Solid Edge part; units mm, degrees
sketch "Sketch1" plane through (0, 0, 0) normal (0, 0, 1) x (1, 0, 0)
  line L0 (-12.5, -3) -> (12.5, -3)
  line L1 (12.5, -3) -> (12.5, 3)
  line L2 (12.5, 3) -> (-12.5, 3)
  line L3 (-12.5, 3) -> (-12.5, -3)
  dimension "D1" = 12.5
  dimension "D2" = 12.5
extrude "Protrusion1" add sketch "Sketch1" along normal blind 2
sketch "Sketch2" plane through (0, 0, 2) normal (0, 0, 1) x (1, 0, 0)
  line L0 (-12.5, 3) -> (12.5, 3)
  line L1 (12.5, 3) -> (12.5, 2)
  line L2 (12.5, 2) -> (-12.5, 2)
  line L3 (-12.5, 2) -> (-12.5, 3)
  line L4 (-12.5, -3) -> (12.5, -3)
  line L5 (12.5, -3) -> (12.5, -1)
  line L6 (12.5, -1) -> (-12.5, -1)
  line L7 (-12.5, -1) -> (-12.5, -3)
  dimension "D1" = 12.5
  dimension "D2" = 12.5
extrude "Extrusionsausprägung_2" add sketch "Sketch2" along normal blind 4
chamfer "Fase_1" distance 0.5 angle 45 3 edges at (0, -3, 6) (0, -1, 6) (0, 2, 6)
Model file for the job. Use its own axes, mm. A direction names the side the tool comes from. Give positions to 0.01 mm unless a question says otherwise; leave off trailing zeros. Write each loop counter-clockwise with the first axis right and the second up, starting at its lowest first coordinate (ties: lowest second). Pieces come first, ordered by that corner, then holes. Notation, with made-up numbers: M 64,41 L 82,41 A21 ccw 82,71 Z; hole C 7,89.25 d9. An arc over 180 degrees is marked long. Use a Markdown table: item, result.
1) Pin check, flat tips, straight feed: pin 1 (1.5 mm diameter, centred on x = 8, y = 2, fed in from -Z); pin 2 (1.5 mm diameter, centred on x = 5, y = 0.5, fed in from +Z). Stop position of each tip, or through.
Responses:
| item | result |
|---|---|
| pin 1 | stops at z = 0 |
| pin 2 | stops at z = 2 |
2) Cut at A-A (z = 4.9). List the corners of the cut face in (x, y).
Responses:
| item | result |
|---|---|
| outline | M -12.5,-3 L 12.5,-3 L 12.5,-1 L -12.5,-1 Z; M -12.5,2 L 12.5,2 L 12.5,3 L -12.5,3 Z |
3) Cut at C-C (y = -0.3). List the corners of the cut face in (x, z).
Responses:
| item | result |
|---|---|
| outline | M -12.5,0 L 12.5,0 L 12.5,2 L -12.5,2 Z |
4) Pull direction Y, two halves, no side cores. Call faces 1 (the flat face through (0, 1, 2)), 2 (the flat face through (0, -2, 6)), 3 (the flat face through (0, -3, 3)): +Y half, -Y half, draft (parallel to the pull), parting line (faces both ways), or undercut.
Responses:
| item | result |
|---|---|
| face 1 | undercut |
| face 2 | draft |
| face 3 | -Y half |
5) Drill centre lines: line 1 (Y direction, x = -1.5, z = 3.15); line 2 (Z direction, x = -10.5, y = -0.6); line 3 (Z direction, x = -10.75, y = 2.3). Where is each one in solid material? Low to high. Write a range as from..to.
Responses:
| item | result |
|---|---|
| line 1 | y = -3..-1, 2..3 |
| line 2 | z = 0..2 |
| line 3 | z = 0..5.8 |
6) Tool access for faces 4 (the flat face through (0, 0, 0)), 5 (the flat face through (0, 2, 4)): list every direction of +Z, -Z, +X, -X, +Y, -Y with a clear straight run to the whole face (end or side of a thin tool).
Responses:
| item | result |
|---|---|
| face 4 | -Z, +X, -X, +Y, -Y |
| face 5 | +Z, +X, -X |
7) Cut at B-B (x = -4.5). List the corners of the cut face in (y, z).
Responses:
| item | result |
|---|---|
| outline | M -3,0 L 3,0 L 3,6 L 2.5,6 L 2,5.5 L 2,2 L -1,2 L -1,5.5 L -1.5,6 L -2.5,6 L -3,5.5 Z |
